Geometry check sheet. Reference: drawing and pictorial views, mm from the part's lowest x, y, z. Give positions to 0.01 mm unless a question says otherwise; leave off trailing zeros. Order: outer loops, then holes, each group sorted by start corner. A loop starts at its lowest first (then second) coordinate and runs counter-clockwise, first axis right, second up.
Item 1: Release check for a two-part mould opening along X. For the marked faces 1, 2 and 3 record: released by +X, released by -X, zero draft, split by the parting line, or undercut.
Item 2: Sectioned sample at B-B on x = 2. Record the boundary of the cut face in (y, z) (1 decimal), and give its area (3 significant figures).
Item 3: Gauge pin test, flat ends, axial feed: P1, Ø1, axis at x = 2.5, z = 11, coming from the +Y side (1 decimal); P2, Ø1, axis at x = 4.5, y = 5.5, coming from the -Z side; P3, Ø3, axis at x = 1.5, z = 8.5, coming from the -Y side. Record the tip position at first contact, or that the pin passes through.
Item 4: Sectioned sample at A-A on x = 4.25. Record the boundary of the cut face in (y, z) (1 decimal).
Item 5: Material ranges on line 1 along X through (y, z) = (19, 4.5); line 2 along Z through (x, y) = (5.75, 15) (1 decimal); line 3 along Y through (x, z) = (3.75, 16) (1 decimal), recorded low to high.
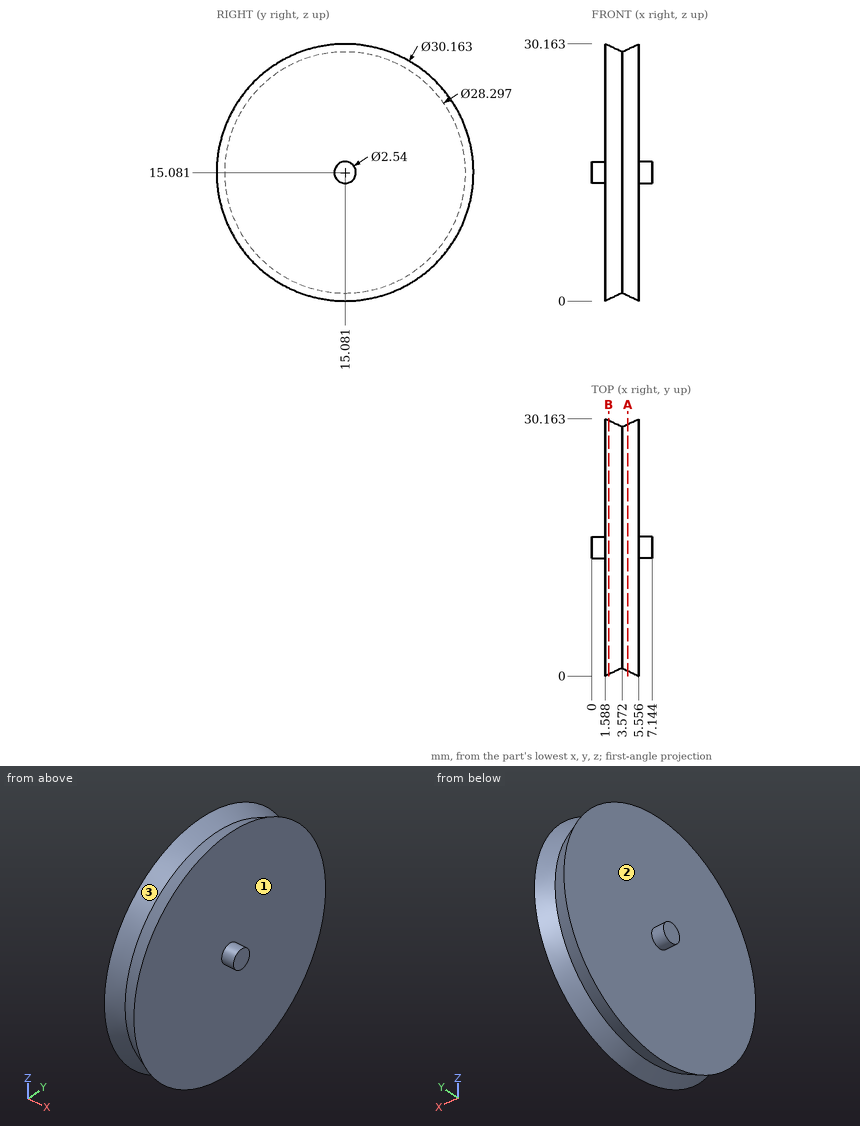
Report:
1. face 1: released by +X
1. face 2: released by -X
1. face 3: undercut
2. outline: circle Ø29.8 at (15.1, 15.1)
2. area: 696 mm2
3. P1: stops at y = 29.4
3. P2: stops at z = 3.57
3. P3: stops at y = 0.88
4. outline: circle Ø28.9 at (15.1, 15.1)
5. line 1: x = 1.59 to 5.56
5. line 2: z = 13.8 to 16.3
5. line 3: y = 0.9 to 29.3
